Source: CAD feature listing. Evaluate the final solid. Frame: model axes, mm. A direction names the side the tool comes from. Give positions to 0.01 mm unless a question says otherwise; leave off trailing zeros. Order: outer loops, then holes, each group sorted by start corner. A loop starts at its lowest first (then second) coordinate and runs counter-clockwise, first axis right, second up. Notation, with made-up numbers: (50.5, 81.5) -> (54.5, 81.5) arc R21 ccw to (54.5, 102.5) -> close; hole circle Ø7 at (67, 18). An arc over 180 degrees is marked (long way). Use CSV: the item, a comma, the result in double quotes.
Autodesk Inventor part; units mm, degrees
ref_plane "Work Plane1" through (10, 0, 42.5) normal (0, 0, -1) x (-1, 0, 0)
ref_plane "Work Plane2" through (0, 0, 22.5) normal (0, 0, 1) x (1, 0, 0)
ref_plane "YZ Plane" through (0, 0, 0) normal (1, 0, 0) x (0, 1, 0)
sketch "Sketch1" plane through (0, 0, 0) normal (0, 1, 0) x (-1, 0, 0)
  line L0 (0, 0) -> (-5, 0)
  line L1 (-5, 0) -> (-5, 45)
  line L2 (-5, 45) -> (0, 45)
  line L3 (0, 45) -> (0, 0)
  line L4 (-5, 45) -> (-20, 45)
  line L5 (-20, 45) -> (-20, 40)
  line L6 (-20, 40) -> (-5, 40)
  line L7 (-5, 40) -> (-5, 45)
  line L8 (-5, 0) -> (-20, 0)
  line L9 (-20, 0) -> (-20, 5)
  line L10 (-20, 5) -> (-5, 5)
  line L11 (-5, 5) -> (-5, 0)
  point P0 (-5, 40)
  point P1 (-5, 5)
  dimension "d0" = 5
  dimension "d1" = 5
  dimension "d2" = 5
  dimension "d3" = 15
  dimension "d4" = 15
  dimension "d5" = 35
extrude "Extrusion1" add sketch "Sketch1" along normal blind 20
sketch "Sketch2" plane through (0, 0, 45) normal (0, 0, 1) x (1, 0, 0)
  circle A0 centre (10, 10) radius 1.75
  line L0 (20, 0) -> (20, 20)
  line L1 (20, 0) -> (10, 0)
  line L2 (10, 0) -> (10, 20)
  line L3 (10, 20) -> (20, 20)
  line L4 (20, 20) -> (20, 0)
  line L5 (0, 0) -> (20, 0)
  dimension "d8" = 10
  dimension "d9" = 10
  dimension "d10" = 10
  dimension "d11" = 3.5
extrude "Extrusion2" cut sketch "Sketch2" against normal blind 200
sketch "Sketch3" plane through (0, 0, 0) normal (-1, 0, 0) x (0, 0, 1)
  line L0 (5, 0) -> (5, 20)
  line L1 (40, 0) -> (40, 20)
  line L2 (5, 15) -> (40, 15)
  line L3 (40, 15) -> (40, 5)
  line L4 (40, 5) -> (5, 5)
  line L5 (5, 5) -> (5, 15)
  line L6 (0, 20) -> (45, 20)
  line L7 (0, 0) -> (45, 0)
  point P0 (5, 5)
  dimension "d14" = 5
  dimension "d15" = 5
extrude "Extrusion3" cut sketch "Sketch3" against normal blind 20 contours L0 L2 L1 L4
sketch "Sketch4" plane through (0, 0, 0) normal (-1, 0, 0) x (0, 0, 1)
  line L0 (45, 0) -> (45, 20)
  line L1 (45, 20) -> (55, 20)
  line L2 (55, 20) -> (55, 0)
  line L3 (55, 0) -> (45, 0)
  line L4 (45, 0) -> (45, 20)
  line L5 (0, 20) -> (0, 11.75)
  line L6 (0, 20) -> (-10, 20)
  line L7 (-10, 20) -> (-10, 0)
  line L8 (-10, 0) -> (0, 0)
  line L9 (0, 0) -> (0, 20)
  circle A0 centre (50, 3) radius 1.375
  circle A1 centre (50, 17) radius 1.375
  circle A2 centre (-5, 17) radius 1.375
  circle A3 centre (-5, 3) radius 1.375
  point P0 (0, 0)
  point P1 (50, 20)
  dimension "d18" = 10
  dimension "d19" = 10
  dimension "d20" = 3
  dimension "d21" = 3
  dimension "d22" = 5
  dimension "d23" = 5
  dimension "d24" = 5
  dimension "d25" = 5
  dimension "d26" = 3
  dimension "d27" = 3
  dimension "d28" = 2.75
  dimension "d29" = 2.75
  dimension "d30" = 2.75
  dimension "d31" = 2.75
extrude "Extrusion4" add sketch "Sketch4" against normal blind 5
sketch "Sketch5" plane through (10, 11.75, 45) normal (1, 0, 0) x (0, 0, -1)
  circle A0 centre (42.5, 5.75) radius 1.35
  circle A1 centre (42.5, -9.25) radius 1.35
  circle A2 centre (2.5, 5.75) radius 1.35
  circle A3 centre (2.5, -9.25) radius 1.35
  line L0 (40, 8.25) -> (45, 8.25)
  line L1 (45, 8.25) -> (45, 0)
  line L2 (45, -3.5) -> (45, -11.75)
  line L3 (45, -11.75) -> (40, -11.75)
  line L4 (5, -11.75) -> (0, -11.75)
  line L5 (0, -11.75) -> (0, -3.5)
  line L6 (0, 0) -> (0, 8.25)
  line L7 (0, 8.25) -> (5, 8.25)
  dimension "d34" = 2.5
  dimension "d35" = 2.5
  dimension "d36" = 2.5
  dimension "d37" = 2.5
  dimension "d38" = 2.5
  dimension "d39" = 2.5
  dimension "d40" = 2.5
  dimension "d41" = 2.5
  dimension "d42" = 2.7
  dimension "d43" = 2.7
  dimension "d44" = 2.7
  dimension "d45" = 2.7
extrude "Extrusion5" cut sketch "Sketch5" against normal blind 15
sketch "Sketch6" plane through (0, 0, 55) normal (-1, 0, 0) x (0, 0, 1)
  circle A0 centre (-12.5, 17.5) radius 1.35
  circle A1 centre (-12.5, 17.5) radius 2
  circle A2 centre (-12.5, 2.5) radius 1.35
  circle A3 centre (-12.5, 2.5) radius 2
  circle A4 centre (-52.5, 2.5) radius 1.35
  circle A5 centre (-52.5, 2.5) radius 2
  circle A6 centre (-52.5, 17.5) radius 1.35
  circle A7 centre (-52.5, 17.5) radius 2
  point P0 (-55, 0)
  dimension "d48" = 4
  dimension "d49" = 4
  dimension "d50" = 4
  dimension "d51" = 4
extrude "Extrusion6" cut sketch "Sketch6" against normal blind 5 contours A0 | A1 | A2 | A3 | A4 | A5 | A6 | A7
ref_plane "Work Plane1" through (10, 0, 42.5) normal (0, 0, -1) x (-1, 0, 0)
sketch "Sketch7" plane through (10, 0, 42.5) normal (0, 0, -1) x (-1, 0, 0)
  line L0 (-3.1754, 10) -> (-1.5877, 12.75)
  line L1 (-1.5877, 12.75) -> (1.5877, 12.75)
  line L2 (1.5877, 12.75) -> (3.1754, 10)
  line L3 (3.1754, 10) -> (1.5877, 7.25)
  line L4 (1.5877, 7.25) -> (-1.5877, 7.25)
  line L5 (-1.5877, 7.25) -> (-3.1754, 10)
  line L6 (0, 11.75) -> (0, 20)
  line L7 (5, 20) -> (0, 20)
  line L8 (5, 0) -> (0, 0)
  point P0 (10, 0)
  point P1 (0, 10)
  dimension "d54" = 2.75
  dimension "d55" = 0
  dimension "d56" = 10
  dimension "d57" = 20
extrude "Extrusion7" cut sketch "Sketch7" along normal mid plane 1.8
ref_plane "Work Plane2" through (0, 0, 22.5) normal (0, 0, 1) x (1, 0, 0)
mirror "Mirror1" about plane through (0, 0, 22.5) normal (0, 0, 1) of "Extrusion7"
equation "\"d14\" = d15"
equation "\"d19\" = d18"
equation "\"d20\" = d21"
equation "\"d24\" = d23"
equation "\"d25\" = d22"
equation "\"d26\" = d20"
equation "\"d27\" = d21"
equation "\"d34\" = d35"
equation "\"d37\" = d34"
equation "\"d38\" = d34"
equation "\"d39\" = d36"
equation "\"d40\" = d39"
equation "\"d41\" = d34"
equation "\"d43\" = d42"
equation "\"d44\" = d42"
equation "\"d45\" = d43"
equation "\"d49\" = d48"
equation "\"d50\" = d49"
equation "\"d51\" = d48"
properties part number "MotorDifferentialMountingBracket"
1. Access query for faces 4 (the flat face through (2, 10, -10)), 5 (the flat face through (5, 10, -5)), 6 (the flat face through (5, 2, 22)), 7 (the flat face through (7.63, 8.606, 2.487)), 8 (the flat face through (5, 1, 3)). Directions: +Z, -Z, +X, -X, +Y, -Y. A direction counts if a zero-diameter tool reaches every point of the face in a straight line with its end or side. Return the directions, or none.
Answer below:
face 4,"-Z, +X, -X, +Y, -Y"
face 5,"-Z, +X, +Y, -Y"
face 6,"+X, +Y, -Y"
face 7,"+X"
face 8,"-X"
2. Section query A-A on x = 5.75. Return loops of the section in (y, z), plus the area to 3 significant figures.
Answer below:
outline,"(0, 0) -> (20, 0) -> (20, 5) -> (0, 5) -> close; (0, 40) -> (20, 40) -> (20, 45) -> (0, 45) -> close; hole circle Ø2.7 at (2.5, 2.5); hole circle Ø2.7 at (2.5, 42.5); hole circle Ø2.7 at (17.5, 2.5); hole circle Ø2.7 at (17.5, 42.5)"
area,"177 mm²"
3. Section query D-D on z = 15. Return loops of the section in (x, y).
Answer below:
outline,"(0, 0) -> (5, 0) -> (5, 5) -> (0, 5) -> close; (0, 15) -> (5, 15) -> (5, 20) -> (0, 20) -> close"
4. Section query B-B on z = 50. Return loops of the section in (x, y) (3 decimals), plus the area to 3 significant figures.
Answer below:
outline,"(0, 0) -> (5, 0) -> (5, 1.625) -> (0, 1.625) -> close; (0, 4.375) -> (5, 4.375) -> (5, 15.625) -> (0, 15.625) -> close; (0, 18.375) -> (5, 18.375) -> (5, 20) -> (0, 20) -> close"
area,"72.5 mm²"
5. Section query C-C on y = 6. Return loops of the section in (x, z).
Answer below:
outline,"(0, -10) -> (5, -10) -> (5, 0) -> (10, 0) -> (10, 5) -> (0, 5) -> close; (0, 40) -> (10, 40) -> (10, 45) -> (5, 45) -> (5, 55) -> (0, 55) -> close"
6. Ray query, line 1 along Y through (x, z) = (6.2, 2.5); line 2 along Y through (x, z) = (2.15, -5) (3 decimals); line 3 along Z through (x, y) = (6.25, 16). Return the intervals inside material, ascending.
Answer below:
line 1,"y = 0 to 1.15, 3.85 to 16.15, 18.85 to 20"
line 2,"y = 0 to 1.625, 4.375 to 15.625, 18.375 to 20"
line 3,"z = 0 to 5, 40 to 45"
7. Pin query (flat end, axial travel): P1, Ø2.5, axis at y = 3, z = 21, coming from the +X side; P2, Ø1.2, axis at y = 17.5, z = 43, coming from the -X side; P3, Ø1, axis at x = 8, y = 15.5, coming from the +Z side; P4, Ø3, axis at y = 2.5, z = 2.5, coming from the -X side. Return the tip coordinate at first contact, or that it passes through.
Answer below:
P1,"stops at x = 5"
P2,"passes through"
P3,"stops at z = 45"
P4,"stops at x = 5"
8. Mould query, pull axis Z, two halves, no side actions, for faces 1 (the cylindrical face through (2.465, 3.06, 48.626)), 2 (the flat face through (10, 4, 3)), 3 (the flat face through (7, 10, 0)). Classes: released by +Z, released by -Z, zero draft, split by the parting line, or undercut.
Answer below:
face 1,"undercut"
face 2,"zero draft"
face 3,"released by -Z"
